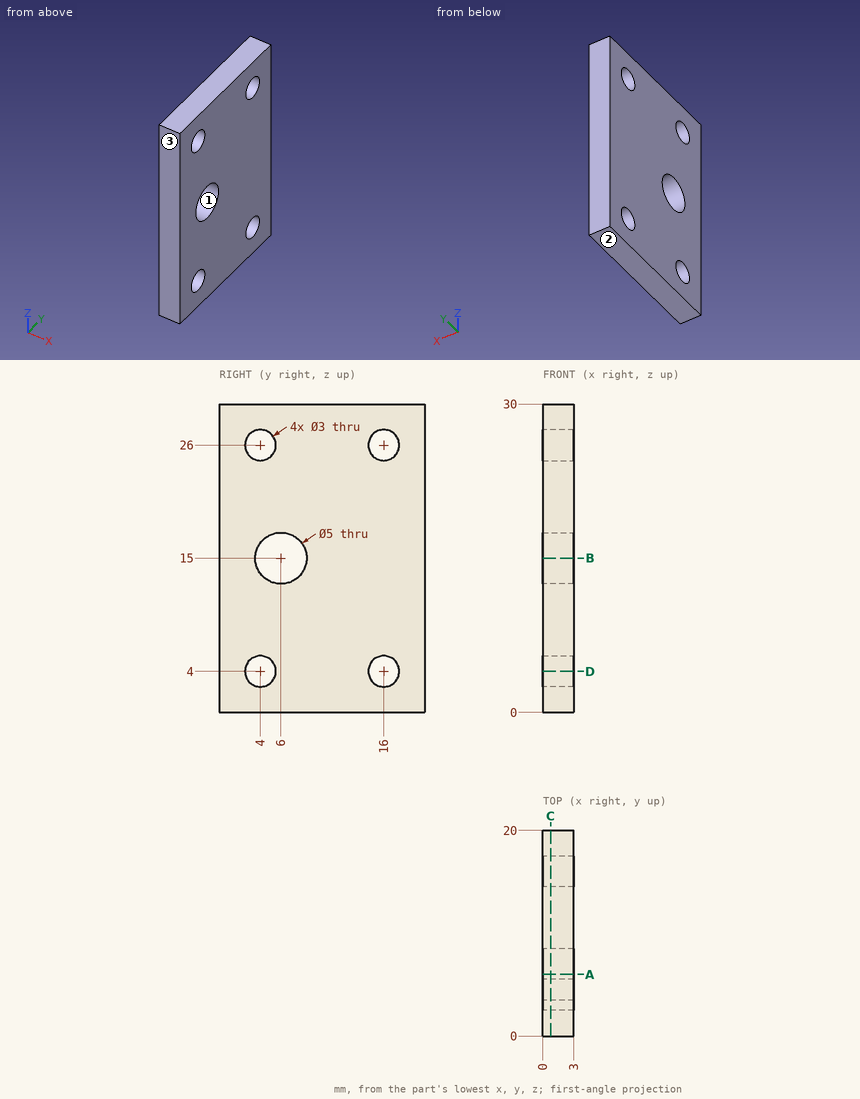
Here's the drawing with two shaded views (mm, measured from the low corner). I have some questions. Round coordinates to 2 decimals unless told otherwise and drop trailing zeros. Loops run counter-clockwise (first coordinate to the right, second up) from the corner with the lowest first, then second, coordinate; pieces in that order, holes last.
Item 1: Suppose I cut it at A-A, the plane y = 6. Write out the boundary of the cut face in (x, z).
Item 2: Will this pin go through, and if not, where does the flat tip stop? pin 1 Ø4 at (y, z) = (6, 15) entering from -X.
Item 3: Suppose I cut it at C-C, the plane x = 0.75. Write out the boundary of the cut face in (y, z).
Item 4: If we mould it in two halves opening along Y, with no side actions, what happens to the marked faces 1, 2 and 3? For each: +Y half, -Y half, draft (parallel to the pull), parting line (faces both ways), or undercut.
Item 5: Please list where these lines run through material, in increasing order: L1, parallel to Y at x = 1.1, z = 26; L2, parallel to Z at x = 2.05, y = 5; L3, parallel to Z at x = 1.8, y = 3.75.
Item 6: Suppose I cut it at D-D, the plane z = 4. Write out the boundary of the cut face in (x, y).
Item 7: Suppose I cut it at B-B, the plane z = 15. Write out the boundary of the cut face in (x, y).
Reported:
1. outline: (0, 0) - (3, 0) - (3, 12.5) - (0, 12.5) - close; (0, 17.5) - (3, 17.5) - (3, 30) - (0, 30) - close
2. pin 1: passes through
3. outline: (0, 0) - (20, 0) - (20, 30) - (0, 30) - close; hole circle Ø3 at (4, 4); hole circle Ø3 at (4, 26); hole circle Ø5 at (6, 15); hole circle Ø3 at (16, 4); hole circle Ø3 at (16, 26)
4. face 1: undercut
4. face 2: draft
4. face 3: -Y half
5. L1: y = 0 to 2.5, 5.5 to 14.5, 17.5 to 20
5. L2: z = 0 to 2.88, 5.12 to 12.71, 17.29 to 24.88, 27.12 to 30
5. L3: z = 0 to 2.52, 5.48 to 13.91, 16.09 to 24.52, 27.48 to 30
6. outline: (0, 0) - (3, 0) - (3, 2.5) - (0, 2.5) - close; (0, 5.5) - (3, 5.5) - (3, 14.5) - (0, 14.5) - close; (0, 17.5) - (3, 17.5) - (3, 20) - (0, 20) - close
7. outline: (0, 0) - (3, 0) - (3, 3.5) - (0, 3.5) - close; (0, 8.5) - (3, 8.5) - (3, 20) - (0, 20) - close
